from build123d import *

# Parameters (mm, degrees)
EXTRUDE_1_DEPTH     = 10
FILLET_1_R          = 10
FILLET_11_R         = 5
FILLET_21_R         = 15
FILLET_24_R         = 11
SKETCH_5_R          = 1.5
CUT_EXTRUDE_1_DEPTH = 6
SKETCH_2_R          = 1.5
CUT_EXTRUDE_2_DEPTH = 6
CUT_EXTRUDE_START   = -6
SKETCH_3_R          = 1.5
CUT_EXTRUDE_3_DEPTH = 6
SKETCH_4_R          = 1.5
CUT_EXTRUDE_4_DEPTH = 6


with BuildPart() as part:
    # 草图1 → 凸台-拉伸1 (new body)
    with BuildSketch(Plane(origin=(0, 0, 0), x_dir=(1, 0, 0), z_dir=(0, 1, 0))):
        Polygon((73.431457505, 42.5), (16.568542495, 42.5), (-17.604076401, 42.5), (-42.5, 17.604076401), (-42.5, -17.604076401), (-17.604076401, -42.5), (16.568542495, -42.5), (73.431457505, -42.5), (107.604076401, -42.5), (132.5, -17.604076401), (132.5, 17.604076401), (107.604076401, 42.5), align=None)
        Polygon((-37.5, 15.533008589), (-29.033008589, 24), (-7.5, 24), (-7.5, -37.5), (-15.533008589, -37.5), (-37.5, -15.533008589), align=None, mode=Mode.SUBTRACT)
        Polygon((19.068542495, -37.5), (16.568542495, -37.5), (6.858116823, -37.5), (-2.5, -37.5), (-2.5, -28), (-2.5, 12.5), (92.5, 12.5), (92.5, -28), (92.5, -37.5), (83.141883177, -37.5), (73.431457505, -37.5), align=None, mode=Mode.SUBTRACT)
        Polygon((97.5, 24), (119.033008589, 24), (127.5, 15.533008589), (127.5, -15.533008589), (105.533008589, -37.5), (97.5, -37.5), align=None, mode=Mode.SUBTRACT)
    extrude(amount=EXTRUDE_1_DEPTH)

    # 圆角1
    fillet_1_edges = [part.edges().sort_by_distance(p)[0] for p in [
        (-7.5, 5, -24),
        (97.5, 5, -24),
    ]]
    fillet(fillet_1_edges, radius=FILLET_1_R)

    # 圆角11
    fillet_11_edges = [part.edges().sort_by_distance(p)[0] for p in [
        (-15.533008589, 5, 37.5),
        (-7.5, 5, 37.5),
        (97.5, 5, 37.5),
        (105.533008589, 5, 37.5),
    ]]
    fillet(fillet_11_edges, radius=FILLET_11_R)

    # 圆角21
    fillet_21_edges = [part.edges().sort_by_distance(p)[0] for p in [
        (-29.033008589, 5, -24),
        (119.033008589, 5, -24),
    ]]
    fillet(fillet_21_edges, radius=FILLET_21_R)

    # 圆角24
    fillet_24_edges = [part.edges().sort_by_distance(p)[0] for p in [
        (-37.5, 5, -15.533008589),
        (127.5, 5, -15.533008589),
    ]]
    fillet(fillet_24_edges, radius=FILLET_24_R)

    # 草图5 → 切除-拉伸1 (cut)
    with BuildSketch(Plane.ZY.offset(42.5)):
        with Locations((10, 5)):
            Circle(SKETCH_5_R)
        with Locations((-10, 5)):
            Circle(SKETCH_5_R)
    extrude(amount=-CUT_EXTRUDE_1_DEPTH, mode=Mode.SUBTRACT)

    # 草图2 → 切除-拉伸2 (cut)
    with BuildSketch(Plane(origin=(0, 0, -42.5), x_dir=(-1, 0, 0), z_dir=(0, 0, -1))):
        with Locations((-33.281955929, 5)):
            Circle(SKETCH_2_R)
        with Locations((-13.281955929, 5)):
            Circle(SKETCH_2_R)
        with Locations((6.718044071, 5)):
            Circle(SKETCH_2_R)
        with Locations(Location((-96.718044071, 5, 0), (0, 0, 180))):
            Circle(SKETCH_2_R)
        with Locations(Location((-76.718044071, 5, 0), (0, 0, 180))):
            Circle(SKETCH_2_R)
        with Locations(Location((-56.718044071, 5, 0), (0, 0, 180))):
            Circle(SKETCH_2_R)
    extrude(amount=-CUT_EXTRUDE_2_DEPTH, mode=Mode.SUBTRACT)

    # 草图3 → 切除-拉伸3 (cut)
    with BuildSketch(Plane(origin=(132.5, 0, 0), x_dir=(0, 0, -1), z_dir=(1, 0, 0)).offset(CUT_EXTRUDE_START)):
        with Locations(Location((10, 5, 0), (0, 0, 180))):
            Circle(SKETCH_3_R)
        with Locations(Location((-10, 5, 0), (0, 0, 180))):
            Circle(SKETCH_3_R)
    extrude(amount=CUT_EXTRUDE_3_DEPTH, mode=Mode.SUBTRACT)

    # 草图4 → 切除-拉伸4 (cut)
    with BuildSketch(Plane.XY.offset(42.5).offset(CUT_EXTRUDE_START)):
        with Locations((56.718044071, 5)):
            Circle(SKETCH_4_R)
        with Locations((76.718044071, 5)):
            Circle(SKETCH_4_R)
        with Locations((96.718044071, 5)):
            Circle(SKETCH_4_R)
        with Locations(Location((33.281955929, 5, 0), (0, 0, 180))):
            Circle(SKETCH_4_R)
        with Locations(Location((13.281955929, 5, 0), (0, 0, 180))):
            Circle(SKETCH_4_R)
        with Locations(Location((-6.718044071, 5, 0), (0, 0, 180))):
            Circle(SKETCH_4_R)
    extrude(amount=CUT_EXTRUDE_4_DEPTH, mode=Mode.SUBTRACT)


solid = part.part
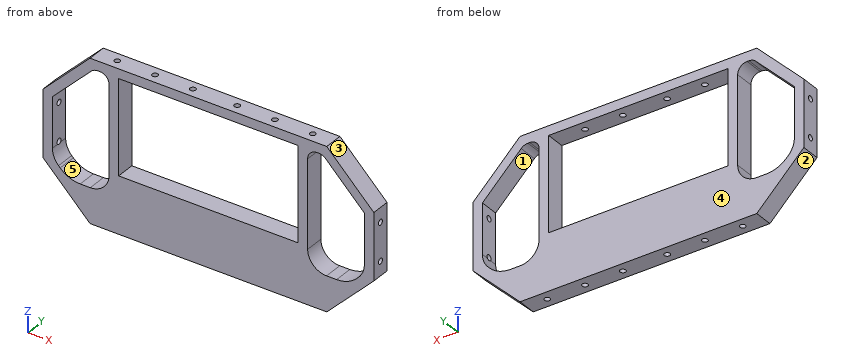
Here's how the part is built. I have some questions about the finished solid (model axes, mm). Face numbers are marked on the shaded views. A direction names the side the tool comes from. Coordinates: 2 decimals unless noted, no trailing zeros. Order: outer loops, then holes, each group sorted by start corner. A loop starts at its lowest first (then second) coordinate and runs counter-clockwise, first axis right, second up. Notation, with made-up numbers: (48, 5) - (80, 5) arc R21 ccw to (80, 14) - close; hole circle Ø11 at (-39, -33.75). An arc over 180 degrees is marked (long way). Use CSV: the item, a comma, the result in double quotes. Start each with the question number.
1. Suppose I cut it at B-B on x = 7.5. List the corners of the cut face in (y, z) for me.
2. Suppose I cut it at C-C on x = 100. List the corners of the cut face in (y, z) for me.
3. Suppose I cut it at A-A on z = 2.5. List the corners of the cut face in (x, y) for me.
4. For the marked faces 1 and 2, which set-ups out of +Z, -Z, +X, -X, +Y, -Y let a thin tool reach every point of the face, with its end or its side?
5. Suppose I cut it at D-D on z = 20.5. List the corners of the cut face in (x, y) for me.
6. Please list where these lines run through material, in increasing order: line 1 (X direction, y = 4.5, z = -1.5); line 2 (Z direction, x = 61.5, y = 8.25); line 3 (X direction, y = 8.5, z = 28.5). Write a range as from..to.
7. I'm going to push flat-ended pins straight in: pin 1 (12 mm diameter, centred on x = 65, z = -9.5, fed in from +Y); pin 2 (2.5 mm diameter, centred on x = -6.72, y = 5, fed in from +Z); pin 3 (3 mm diameter, centred on y = 4, z = 24.5, fed in from -X); pin 4 (2.5 mm diameter, centred on x = 56.72, y = 5, fed in from +Z). Where does each tip first touch, or does it pass through?
8. If we mould it in two halves opening along X, with no side actions, what happens to the marked faces 3, 4 and 5? For each: +X half, -X half, draft (parallel to the pull), parting line (faces both ways), or undercut.
Output:
1,outline,"(0, -42.5) - (10, -42.5) - (10, -12.5) - (0, -12.5) - close; (0, 37.5) - (10, 37.5) - (10, 42.5) - (0, 42.5) - close"
2,outline,"(0, -42.5) - (10, -42.5) - (10, -20.61) - (0, -20.61) - close; (0, 36.83) - (10, 36.83) - (10, 42.5) - (0, 42.5) - close"
3,outline,"(-42.5, 0) - (-37.5, 0) - (-37.5, 10) - (-42.5, 10) - close; (-7.5, 0) - (-2.5, 0) - (-2.5, 10) - (-7.5, 10) - close; (92.5, 0) - (97.5, 0) - (97.5, 10) - (92.5, 10) - close; (127.5, 0) - (132.5, 0) - (132.5, 10) - (127.5, 10) - close"
4,face 1,"+Y, -Y"
4,face 2,"-Z, -X, +Y, -Y"
5,outline,"(-39.6, 0) - (-32.53, 0) - (-32.53, 10) - (-39.6, 10) - close; (-7.5, 0) - (-2.5, 0) - (-2.5, 10) - (-7.5, 10) - close; (92.5, 0) - (97.5, 0) - (97.5, 10) - (92.5, 10) - close; (122.53, 0) - (129.6, 0) - (129.6, 10) - (122.53, 10) - close"
6,line 1,"x = -42.5..-37.5, -7.5..-2.5, 92.5..97.5, 127.5..132.5"
6,line 2,"z = -42.5..-12.5, 37.5..42.5"
6,line 3,"x = -31.6..-24.53, -7.5..-2.5, 92.5..97.5, 114.53..121.6"
7,pin 1,"stops at y = 10"
7,pin 2,"stops at z = 36.5"
7,pin 3,"stops at x = -37.1"
7,pin 4,"stops at z = -12.5"
8,face 3,"+X half"
8,face 4,"draft"
8,face 5,"undercut"
